Design review of the part built by this model. Coordinates are the model's own, in mm. A direction names the side the tool comes from. Give positions to 0.01 mm unless a question says otherwise; leave off trailing zeros. Loops run counter-clockwise (first coordinate to the right, second up) from the corner with the lowest first, then second, coordinate; pieces in that order, holes last. Notation, with made-up numbers: (52.5, 2) -> (84.5, 2) arc R16 ccw to (84.5, 6) -> close; hole circle Ø5 at (28.5, 19). An arc over 180 degrees is marked (long way). Use CSV: the item, a comma, the result in double quotes. Start each with the question number.
Item 1: The part is to be moulded in two halves that separate along X. For faces 1 (the face through (0, 16, -2)), 2 (the face through (-6.09, 14.55, 3.94)), 3 (the face through (8.132, 15.975, 3.07)), 4 (the face through (-8.163, 15.547, 3.07)), say which applies: +X half, -X half, draft (parallel to the pull), parting line (faces both ways), or undercut.
Item 2: Wall thickness on line 1 along Y through (x, z) = (-2.5, 5.75); line 2 along Z through (x, y) = (-4, 16); line 3 along X through (y, z) = (20, 7.25): over which ranges is each line inside the solid? List them lowest first. Write a range as from..to.
Item 3: Clearance check with flat-ended pins moving along their axes: pin 1 (4 mm diameter, centred on x = 2, z = 2.5, fed in from -Y); pin 2 (2 mm diameter, centred on y = 3.5, z = 6.5, fed in from +X); pin 3 (7 mm diameter, centred on x = -1, y = 17.5, fed in from +Z). State where each tip first meets the part, or that it passes through.
Item 4: We need section C-C (y = 6). State the section outline as (x, z) points.
Item 5: We need section D-D (z = -1). State the section outline as (x, y) points.
Item 6: We need section B-B (x = -2.5). State the section outline as (y, z) points, plus the area to 3 significant figures.
Item 7: For faces 5 (the face through (0, 15, 0)), 6 (the face through (6, 18, 8)), list the 3-axis set-ups (+Z, -Z, +X, -X, +Y, -Y) from which the entire face can be reached by the end or side of a thin tool; tool diameter is ignored.
Item 8: We need section A-A (z = 5.75). State the section outline as (x, y) points.
from build123d import *

# Parameters (mm, degrees)
PAD_DEPTH      = 8
PAD_DEPTH_BACK = 2
POCKET_DEPTH   = 8.001
CHAMFER_SIZE   = 0.5


with BuildPart() as part:
    # Sketch001 → Pad (new body, two sides)
    with BuildSketch(Plane.XY) as pad_sk:
        Polygon((-9.295655, 0), (-7, 31.521814), (7, 31.521814), (9.295655, 0), align=None)
    extrude(amount=PAD_DEPTH)
    extrude(pad_sk.sketch, amount=-PAD_DEPTH_BACK)

    # Sketch → Pocket (cut, through all)
    with BuildSketch(Plane.XY):
        Polygon((-7.15, 0), (-5, 29.521814), (5, 29.521814), (7.15, 0), align=None)
    extrude(amount=POCKET_DEPTH, mode=Mode.SUBTRACT)

    # Chamfer
    chamfer_edges = [part.edges().sort_by_distance(p)[0] for p in [
        (7, 31.521814, 3),
        (-7, 31.521814, 3),
        (-9.295655, 0, 3),
        (9.295655, 0, 3),
    ]]
    chamfer(chamfer_edges, length=CHAMFER_SIZE)


solid = part.part
Results found:
1,face 1,"draft"
1,face 2,"undercut"
1,face 3,"+X half"
1,face 4,"-X half"
2,line 1,"29.52..31.52"
2,line 2,"-2..0"
2,line 3,"-7.84..-5.69, 5.69..7.84"
3,pin 1,"y = 29.52"
3,pin 2,"x = 9.11"
3,pin 3,"z = 0"
4,outline,"(-8.86, -2) -> (8.86, -2) -> (8.86, 8) -> (6.71, 8) -> (6.71, 0) -> (-6.71, 0) -> (-6.71, 8) -> (-8.86, 8) -> close"
5,outline,"(-9.26, 0.5) -> (-8.8, 0) -> (8.8, 0) -> (9.26, 0.5) -> (7.04, 31.02) -> (6.5, 31.52) -> (-6.5, 31.52) -> (-7.04, 31.02) -> close"
6,outline,"(0, -2) -> (31.52, -2) -> (31.52, 8) -> (29.52, 8) -> (29.52, 0) -> (0, 0) -> close"
6,area,"79.0 mm²"
7,face 5,"+Z, -Y"
7,face 6,"+Z, +X, -X, +Y, -Y"
8,outline,"(-9.26, 0.5) -> (-8.8, 0) -> (-7.15, 0) -> (-5, 29.52) -> (5, 29.52) -> (7.15, 0) -> (8.8, 0) -> (9.26, 0.5) -> (7.04, 31.02) -> (6.5, 31.52) -> (-6.5, 31.52) -> (-7.04, 31.02) -> close"
